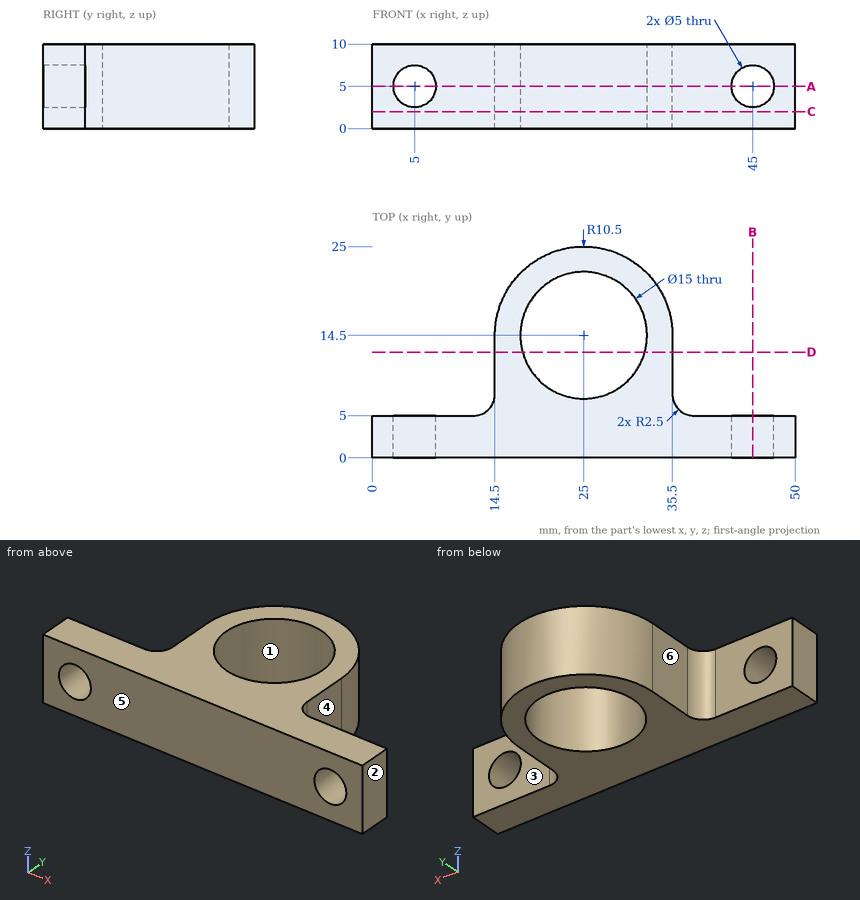
Design review of the part shown in the three views and the two pictorial views. Dimensions are in mm from the part's minimum x, y and z. A direction names the side the tool comes from. Round coordinates to 2 decimals unless told otherwise and drop trailing zeros. Write each loop counter-clockwise with the first axis right and the second up, starting at its lowest first coordinate (ties: lowest second). Pieces come first, ordered by that corner, then holes. Notation, with made-up numbers: (22, 71) - (40, 71) arc R27 ccw to (40, 94) - close; hole circle Ø10 at (1, 29.25). An arc over 180 degrees is marked (long way). Return JSON: item names as keys, results as strings. Group by question number.
Item 1: We need section B-B on x = 45. Write out the cut boundary in (y, z), and give its area (3 significant figures).
Item 2: For probe 1 along X at (y, z) = (2.4, 5); probe 2 along Y at (x, z) = (25, 2.75); probe 3 along Y at (x, z) = (19.5, 8.25), list the stretches that pass through material, from the lowest coordinate up. Write a range as [from, to].
Item 3: We need section D-D on y = 12.5. Write out the cut boundary in (x, z).
Item 4: We need section A-A on z = 5. Write out the cut boundary in (x, y), and give its area (3 significant figures).
Item 5: Insertion check: P1, Ø5, axis at x = 5.5, z = 6, coming from the +Y side; P2, Ø10, axis at x = 8.5, y = 20, coming from the +Z side; P3, Ø5.5, axis at y = 12, z = 3, coming from the -X side; P4, Ø10, axis at x = 33, y = 14, coming from the -Z side. Each pin has a flat end and moves straight along its axis. Give the tip position at first contact, or say it passes through.
Item 6: We need section C-C on z = 2. Write out the cut boundary in (x, y), and give its area (3 significant figures).
Item 7: Machinability: for the marked faces 4, 5 and 6, which of the approach directions +Z, -Z, +X, -X, +Y, -Y give a long, thin tool a straight path to every point of the face, cutting with its end or side? Answer none if there is none.
Item 8: The part is to be moulded in two halves that separate along Y. For the marked faces 1, 2 and 3, say which applies: pulls with the +Y half, pulls with the -Y half, needs draft (parallel to the pull), parting line crosses it, or undercut.
Model answer:
{
 "1": {"outline": "(0, 0) - (5, 0) - (5, 2.5) - (0, 2.5) - close; (0, 7.5) - (5, 7.5) - (5, 10) - (0, 10) - close", "area": "25.0 mm²"},
 "2": {"probe 1": "x = [0, 2.5], [7.5, 42.5], [47.5, 50]", "probe 2": "y = [0, 7], [22, 25]", "probe 3": "y = [0, 9.4], [19.6, 23.44]"},
 "3": {"outline": "(14.5, 0) - (17.77, 0) - (17.77, 10) - (14.5, 10) - close; (32.23, 0) - (35.5, 0) - (35.5, 10) - (32.23, 10) - close"},
 "4": {"outline": "(0, 0) - (2.5, 0) - (2.5, 5) - (0, 5) - close; (7.5, 0) - (42.5, 0) - (42.5, 5) - (38, 5) arc R2.5 cw to (35.5, 7.5) - (35.5, 14.5) arc R10.5 ccw to (14.5, 14.5) - (14.5, 7.5) arc R2.5 cw to (12, 5) - (7.5, 5) - close; (47.5, 0) - (50, 0) - (50, 5) - (47.5, 5) - close; hole circle Ø15 at (25, 14.5)", "area": "399 mm²"},
 "5": {"P1": "stops at y = 5", "P2": "passes through", "P3": "stops at x = 14.5", "P4": "stops at z = 0"},
 "6": {"outline": "(0, 0) - (50, 0) - (50, 5) - (38, 5) arc R2.5 cw to (35.5, 7.5) - (35.5, 14.5) arc R10.5 ccw to (14.5, 14.5) - (14.5, 7.5) arc R2.5 cw to (12, 5) - (0, 5) - close; hole circle Ø15 at (25, 14.5)", "area": "449 mm²"},
 "7": {"face 4": "+Z, -Z, +X, +Y", "face 5": "+Z, -Z, +X, -X, -Y", "face 6": "+Z, -Z, -X, +Y"},
 "8": {"face 1": "undercut", "face 2": "needs draft", "face 3": "pulls with the +Y half"}
}
